The listing builds one solid part. Answer for the finished solid, in the listing's coordinates (mm). Face numbers are marked on the shaded views. A direction names the side the tool comes from. Give positions to 0.01 mm unless a question says otherwise; leave off trailing zeros. Order: outer loops, then holes, each group sorted by start corner. A loop starts at its lowest first (then second) coordinate and runs counter-clockwise, first axis right, second up. Notation, with made-up numbers: (-23.5, -32.75) - (-5.5, -32.75) arc R20 cw to (-5.5, -9.75) - close; hole circle Ø7 at (66, -20.75). An arc over 180 degrees is marked (long way). Answer in a Markdown table with one row per item.
from build123d import *

# Parameters (mm, degrees)
SKETCH1_W           = 16
SKETCH1_H           = 40
SKETCH1_R           = 2.3
SKETCH1_R_2         = 0.9
BOSS_EXTRUDE1_DEPTH = 2
BOSS_EXTRUDE2_DEPTH = 1.5
BOSS_EXTRUDE3_DEPTH = 1.5
SKETCH4_W           = 16
SKETCH4_H           = 40
SKETCH4_R           = 1.75
BOSS_EXTRUDE4_DEPTH = 1.5


with BuildPart() as part:
    # Sketch1 → Boss-Extrude1 (new body)
    with BuildSketch(Plane(origin=(0, 0, 0), x_dir=(1, 0, 0), z_dir=(0, 1, 0))):
        with Locations((8, 20)):
            Rectangle(SKETCH1_W, SKETCH1_H)
        with Locations((8, 35)):
            Circle(SKETCH1_R, mode=Mode.SUBTRACT)
        with Locations((3.5, 35)):
            Circle(SKETCH1_R_2, mode=Mode.SUBTRACT)
        with Locations((12.5, 35)):
            Circle(SKETCH1_R_2, mode=Mode.SUBTRACT)
    extrude(amount=BOSS_EXTRUDE1_DEPTH)

    # Sketch2 → Boss-Extrude2 (add)
    with BuildSketch(Plane.ZY):
        Polygon((-40, 2), (-30, 12), (0, 12), (0, 2), align=None)
    extrude(amount=-BOSS_EXTRUDE2_DEPTH)

    # Sketch3 → Boss-Extrude3 (add)
    with BuildSketch(Plane(origin=(16, 0, -16), x_dir=(0, 0, 1), z_dir=(-1, 0, 0))):
        Polygon((-24, 2), (-14, 12), (16, 12), (16, 2), align=None)
    extrude(amount=BOSS_EXTRUDE3_DEPTH)

    # Sketch4 → Boss-Extrude4 (add)
    with BuildSketch(Plane.XY):
        with Locations((8, 20)):
            Rectangle(SKETCH4_W, SKETCH4_H)
        with Locations((8, 11.197621249)):
            Circle(SKETCH4_R, mode=Mode.SUBTRACT)
        with Locations((8, 29.249612775)):
            Circle(SKETCH4_R, mode=Mode.SUBTRACT)
    extrude(amount=-BOSS_EXTRUDE4_DEPTH)


solid = part.part
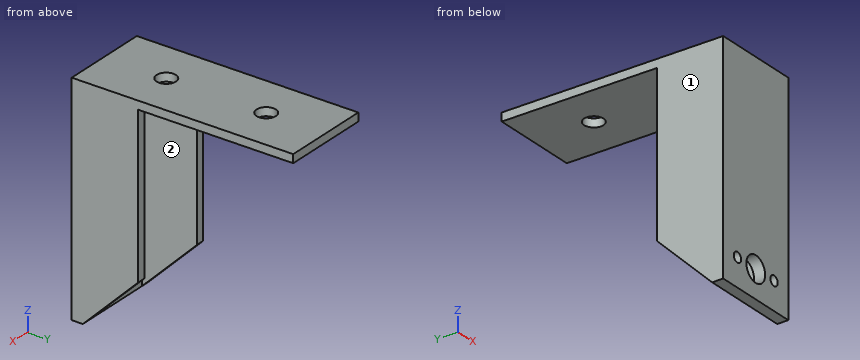
Item 1: Consider line 1 (X direction, y = 1, z = -35); line 2 (Y direction, x = 8, z = -1.1); line 3 (Z direction, x = 8, y = 1). Determine where each line is inside the solid, lowest interval first.
Answer block:
| item | result |
|---|---|
| line 1 | 0 to 2.6, 4.4 to 5.7, 10.3 to 11.6, 13.4 to 16 |
| line 2 | 0 to 9.45, 12.95 to 27.5, 31 to 40 |
| line 3 | -40 to -37.3, -32.7 to 0 |
Item 2: Find section A-A on z = -35. Write down the section's boundary in (x, y), then the cut area to 3 significant figures.
Answer block:
| item | result |
|---|---|
| outline | (0, 0) - (2.6, 0) - (2.6, 2) - (1.5, 2) - (1.5, 7) - (0, 7) - close; (4.4, 0) - (5.7, 0) - (5.7, 2) - (4.4, 2) - close; (10.3, 0) - (11.6, 0) - (11.6, 2) - (10.3, 2) - close; (13.4, 0) - (16, 0) - (16, 7) - (14.5, 7) - (14.5, 2) - (13.4, 2) - close |
| area | 30.6 mm² |
Item 3: Find section B-B on x = 12.5. Write down the section's boundary in (y, z), then the cut area to 3 significant figures.
Answer block:
| item | result |
|---|---|
| outline | (0, -40) - (2, -40) - (2, -35.9) - (0, -35.9) - close; (0, -34.1) - (2, -34.1) - (2, -1.5) - (40, -1.5) - (40, 0) - (0, 0) - close |
| area | 133 mm² |
Item 4: Find section D-D on y = 30. Write down the section's boundary in (x, z), then the cut area to 3 significant figures.
Answer block:
| item | result |
|---|---|
| outline | (0, -1.5) - (6.42, -1.5) - (6.42, 0) - (0, 0) - close; (9.58, -1.5) - (16, -1.5) - (16, 0) - (9.58, 0) - close |
| area | 19.3 mm² |
Item 5: Each of these flat-tipped pins is pushed along its axis until it touches: P1, Ø1, axis at x = 12.5, y = 15, coming from the +Z side; P2, Ø2, axis at x = 8, y = 11.2, coming from the +Z side; P3, Ø4, axis at x = 4.5, z = -8, coming from the +Y side; P4, Ø4, axis at x = 8, y = 29.25, coming from the -Z side. Where does it stop, or does it pass through?
Answer block:
| item | result |
|---|---|
| P1 | z = 0 |
| P2 | through |
| P3 | y = 2 |
| P4 | z = -1.5 |
Item 6: Which of the six approach directions +Z, -Z, +X, -X, +Y, -Y give full straight-line access (tool end or side, diameter ignored) to the marked faces 1 and 2?
Answer block:
| item | result |
|---|---|
| face 1 | +Z, -Z, -X, +Y, -Y |
| face 2 | -Z, +Y |
Item 7: Find section C-C on x = 8. Write down the section's boundary in (y, z).
Answer block:
| item | result |
|---|---|
| outline | (0, -40) - (2, -40) - (2, -37.3) - (0, -37.3) - close; (0, -32.7) - (2, -32.7) - (2, -1.5) - (9.45, -1.5) - (9.45, 0) - (0, 0) - close; (12.95, -1.5) - (27.5, -1.5) - (27.5, 0) - (12.95, 0) - close; (31, -1.5) - (40, -1.5) - (40, 0) - (31, 0) - close |
